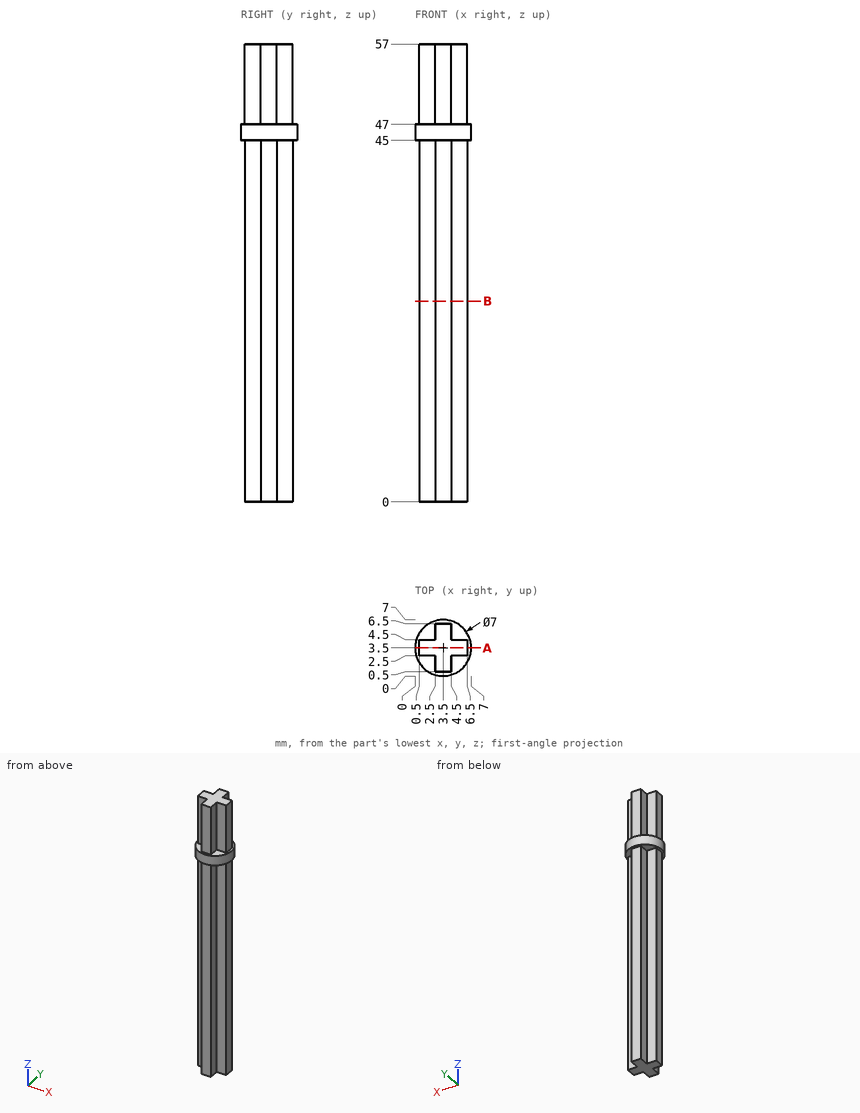
Study the drawing (mm; zero at the part's minimum x, y, z) and answer. Coordinates: 2 decimals unless noted, no trailing zeros. Write each loop counter-clockwise with the first axis right and the second up, starting at its lowest first coordinate (ties: lowest second). Pieces come first, ordered by that corner, then holes. Notation, with made-up numbers: M 24.25,77.25 L 64.25,77.25 A30 ccw 64.25,108.25 Z; hole C 22,-11 d10. An arc over 180 degrees is marked long. Write each question's results on one line, items separated by ' | '.
Item 1: The part is cut by section A-A on y = 3.5. Determine the outline of the cut face in (x, z), and give its area (3 significant figures).
Answer below:
outline: M 0,45 L 0.5,45 L 0.5,0 L 6.5,0 L 6.5,45 L 7,45 L 7,47 L 6.5,47 L 6.5,57 L 0.5,57 L 0.5,47 L 0,47 Z | area: 344 mm2
Item 2: Consider probe 1 along Y at (x, z) = (1, 51.5); probe 2 along Z at (x, y) = (6.5, 1.75). Determine where each line is inside the solid, lowest interval first. Write a range as [from, to].
Answer below:
probe 1: [2.5, 4.5] | probe 2: [45, 47]
Item 3: The part is cut by section B-B on z = 25. Determine the outline of the cut face in (x, y), and give its area (3 significant figures).
Answer below:
outline: M 0.5,2.5 L 2.5,2.5 L 2.5,0.5 L 4.5,0.5 L 4.5,2.5 L 6.5,2.5 L 6.5,4.5 L 4.5,4.5 L 4.5,6.5 L 2.5,6.5 L 2.5,4.5 L 0.5,4.5 Z | area: 20.0 mm2
Item 4: Given P1, Ø2, axis at x = 4.5, z = 44.5, coming from the +Y side; P2, Ø2, axis at y = 2.5, z = 43.5, coming from the -X side; P3, Ø1, axis at y = 1.5, z = 31, coming from the +X side, each flat-ended and moving along its own axis, determine where each tip first touches the part or whether it passes through.
Answer below:
P1: y = 7 | P2: x = 0.5 | P3: x = 4.5
